```python
from build123d import *

# Parameters (mm, degrees)
F0_W     = 135
F0_H     = 180
F1_DEPTH = 25
F3_DEPTH = 180
F4_W     = 51.5650697052
F4_H     = 42.2876738012
F5_DEPTH = 25
F6_W     = 66.04
F6_H     = 31
F7_DEPTH = 25
F8_W     = 32.0292665178
F8_H     = 42.2876738012
F9_DEPTH = 10


# Not quite as in the source:
# - a feature names something its author has since deleted; it is built from what else it names


with BuildPart() as f1:
    # F0 (on Front) → F1 (new body)
    with BuildSketch(Plane.XZ):
        Rectangle(F0_W, F0_H)
    extrude(amount=F1_DEPTH)

    # F2 (on face) → F3 (join)
    with BuildSketch(Plane(origin=(0, 0, -90), x_dir=(1, 0, 0), z_dir=(0, 0, -1))):
        Polygon((-74.269764297, 20.2139050914), (-67.5, 25), (-62.1096342802, 25), (-59.8334595561, 48.8052852452), align=None)
        Polygon((-67.5, 0), (-67.5, 25), (-74.269764297, 20.2139050914), (-102.8616279364, 0), align=None)
    extrude(amount=-F3_DEPTH)

    # F4 (on face) → F5 (cut)
    with BuildSketch(Plane(origin=(-34.2790786746, -48.4865610438, 0), x_dir=(0.8165449841, -0.5772818107, 0), z_dir=(-0.5772818107, -0.8165449841, 0))):
        with Locations((-54.0774967521, 1.7260275781)):
            Rectangle(F4_W, F4_H)
    extrude(amount=-F5_DEPTH, mode=Mode.SUBTRACT)

    # F6 (on face) → F7 (cut)
    with BuildSketch(Plane.XZ.offset(25)):
        with Locations((13.1429424509, 66.5)):
            Rectangle(F6_W, F6_H)
        with Locations((13.1429424509, -66.5)):
            Rectangle(F6_W, F6_H)
    extrude(amount=-F7_DEPTH, mode=Mode.SUBTRACT)

    # F8 (on face) → F9 (cut)
    with BuildSketch(Plane(origin=(-67.3147543785, -33.9884364638, 0), x_dir=(0.4507223021, -0.8926642181, 0), z_dir=(-0.8926642181, -0.4507223021, 0))):
        with Locations((0.5838238992, 1.7260275781)):
            Rectangle(F8_W, F8_H)
    extrude(amount=-F9_DEPTH, mode=Mode.SUBTRACT)


solid = f1.part
```
Geometry: final body of the model. Coordinates: model frame, mm. A direction names the side the tool comes from. Round coordinates to 2 decimals unless told otherwise and drop trailing zeros. Write each loop counter-clockwise with the first axis right and the second up, starting at its lowest first coordinate (ties: lowest second). Pieces come first, ordered by that corner, then holes. Notation, with made-up numbers: (32.25, 21) -> (55.25, 21) arc R33 ccw to (55.25, 58) -> close; hole circle Ø8 at (68, -3). An arc over 180 degrees is marked (long way). Use CSV: the item, a comma, the result in double quotes. Start each with the question number.
Q1. Line query: L1, parallel to Z at x = 10.5, y = -9; L2, parallel to Z at x = -71.5, y = -21; L3, parallel to Y at x = 24, z = -26.5. Output: solid intervals per line, ascending.
Q2. Reachability of faces 1 (the face through (-19.877, -13, 66)), 2 (the face through (0, -14, -90)), 3 (the face through (-60.987, -36.736, -55.203)) from +Z, -Z, +X, -X, +Y, -Y: full face, straight path, thin tool, end or side. Return the list, or none.
Q3. Section A-A (z = 16). Return loops of the section in (x, y).
Q4. Section B-B (x = 29.5). Return loops of the section in (y, z).
Q5. Section C-C (y = -16). Return loops of the section in (x, z).
Q6. First-contact query: pin 1 Ø1 at (x, z) = (-45.5, 5) entering from +Y; pin 2 Ø12.5 at (y, z) = (-10.5, 66.5) entering from -X; pin 3 Ø6 at (x, z) = (-35.5, 33.5) entering from -Y; pin 4 Ø2 at (y, z) = (-24, 45) entering from -X. Flat tips, straight axial feed; report the tip coordinate or a pass-through.
Q7. Pull-direction query (Y, two-part tool) for faces 4 (the face through (-47.704, -18.462, 1.43)), 5 (the face through (-51.369, -5.787, 2.022)), 6 (the face through (13, -13, 82)), 7 (the face through (-66.95, -34.71, 55.97)); classes: pulls with the +Y half, pulls with the -Y half, needs draft (parallel to the pull), parting line crosses it, or undercut.
Q8. Section D-D (x = -92). Return loops of the section in (y, z), plus the area to 3 significant figures.
Result sheet:
1,L1,"-90 to -82, -51 to 51, 82 to 90"
1,L2,"-90 to -19.42, 22.87 to 90"
1,L3,"-25 to 0"
2,face 1,"+Y, -Y"
2,face 2,"-Z, +X, -X, +Y, -Y"
2,face 3,"+Z, -Z, +X"
3,outline,"(-102.86, 0) -> (-99.49, -2.38) -> (-97.8, 0) -> close; (-59.56, 0) -> (-42.95, -11.74) -> (-52.33, -25) -> (67.5, -25) -> (67.5, 0) -> close"
4,outline,"(-25, -90) -> (0, -90) -> (0, -82) -> (-25, -82) -> close; (-25, -51) -> (0, -51) -> (0, 51) -> (-25, 51) -> close; (-25, 82) -> (0, 82) -> (0, 90) -> (-25, 90) -> close"
5,outline,"(-80.23, -90) -> (67.5, -90) -> (67.5, 90) -> (-80.23, 90) -> (-80.23, 22.87) -> (-45.96, 22.87) -> (-45.96, -19.42) -> (-80.23, -19.42) -> close; hole (-19.88, -82) -> (46.16, -82) -> (46.16, -51) -> (-19.88, -51) -> close; hole (-19.88, 51) -> (46.16, 51) -> (46.16, 82) -> (-19.88, 82) -> close"
6,pin 1,"y = 0"
6,pin 2,"x = -96.85"
6,pin 3,"y = -25"
6,pin 4,"x = -72.86"
7,face 4,"undercut"
7,face 5,"undercut"
7,face 6,"needs draft"
7,face 7,"pulls with the -Y half"
8,outline,"(-7.68, -90) -> (0, -90) -> (0, -19.42) -> (-7.68, -19.42) -> close; (-7.68, 22.87) -> (0, 22.87) -> (0, 90) -> (-7.68, 90) -> close"
8,area,"1,060 mm²"
